Could you check a few things on this drawing? It's one solid part, dimensions in mm from its lowest x, y, z. Coordinates: 2 decimals unless noted, no trailing zeros. Write each loop counter-clockwise with the first axis right and the second up, starting at its lowest first coordinate (ties: lowest second). Pieces come first, ordered by that corner, then holes. Notation, with made-up numbers: (51, 40) - (64, 40) arc R21 cw to (64, 67) - close; hole circle Ø2 at (6.5, 0.5). An arc over 180 degrees is marked (long way). Answer as a JSON object with one key per item and string values. Group by question number.
1) If we section it at A-A (y = 97.79): Write out the boundary of the cut face in (x, z) (1 decimal).
2) Please list where these lines run through material, in increasing order: line 1 along Y through (x, z) = (81, 3.7); line 2 along Y through (x, z) = (136.5, 0.9) (1 decimal); line 3 along Y through (x, z) = (29.5, 1.8) (1 decimal).
3) If we section it at D-D (x = 157.5): Write out the boundary of the cut face in (y, z), plus the area to 3 significant figures.
4) Will these pins go through, and if not, where does the flat tip stop? pin 1 Ø1.4 at (x, z) = (46, 2) entering from +Y; pin 2 Ø2.5 at (y, z) = (381, 1.5) entering from -X.
5) If we section it at B-B (z = 2.65): State how many separate pieces and enclosed holes the cut face has, plus the area to 3 significant figures.
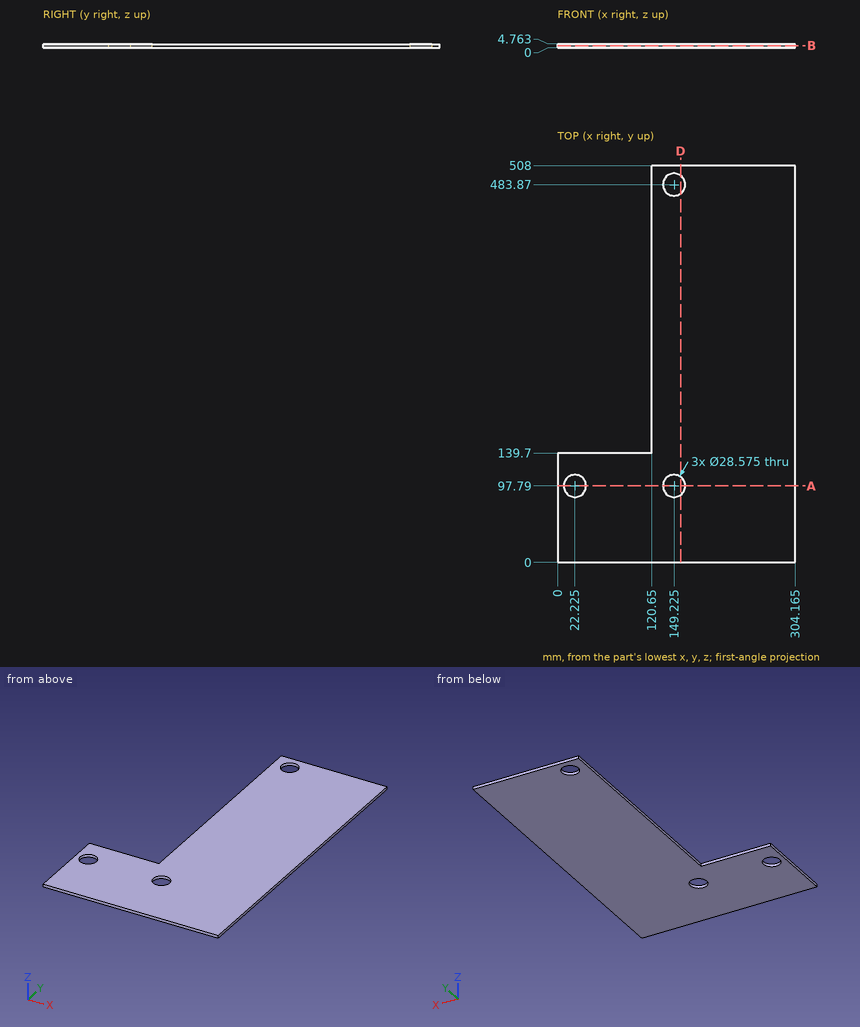
Here are the results:
{
 "1": {"outline": "(0, 0) - (7.9, 0) - (7.9, 4.8) - (0, 4.8) - close; (36.5, 0) - (134.9, 0) - (134.9, 4.8) - (36.5, 4.8) - close; (163.5, 0) - (304.2, 0) - (304.2, 4.8) - (163.5, 4.8) - close"},
 "2": {"line 1": "y = 0 to 139.7", "line 2": "y = 0 to 91.3, 104.3 to 477.4, 490.4 to 508", "line 3": "y = 0 to 85.5, 110.1 to 139.7"},
 "3": {"outline": "(0, 0) - (86.14, 0) - (86.14, 4.76) - (0, 4.76) - close; (109.44, 0) - (472.22, 0) - (472.22, 4.76) - (109.44, 4.76) - close; (495.52, 0) - (508, 0) - (508, 4.76) - (495.52, 4.76) - close", "area": "2,200 mm²"},
 "4": {"pin 1": "stops at y = 139.7", "pin 2": "stops at x = 120.65"},
 "5": {"separate pieces": "1", "enclosed holes": "3", "area": "108,000 mm²"}
}
